Part model, mm, in its own coordinate system. A direction names the side the tool comes from. Round coordinates to 2 decimals unless told otherwise and drop trailing zeros. Write each loop counter-clockwise with the first axis right and the second up, starting at its lowest first coordinate (ties: lowest second). Pieces come first, ordered by that corner, then holes. Notation, with made-up numbers: M 3,61 L 25,61 A26 ccw 25,89 Z; hole C 63,-13 d6. An arc over 180 degrees is marked long. Use one line per item in the form item = value. Start each with the question number.
Item 1: Flat gauge pins, fed straight in: pin 1 Ø12 at (x, z) = (54.5, 4.5) entering from -Y; pin 2 Ø2 at (x, y) = (54, 2) entering from -Z (3 decimals); pin 3 Ø2 at (x, y) = (22.5, -13.5) entering from -Z. Where does each tip first touch, or does it go through?
Item 2: Probe L1, parallel to X at y = -23, z = -4; L2, parallel to X at y = -5, z = 13.5; L3, parallel to Z at x = 27, y = -2. List the from-to ranges inside material, lowest first.
Item 3: Which spindle directions (+Z, -Z, +X, -X, +Y, -Y) get a long thin tool onto all of the face, cutting with end or side? Do faces 1 (the face through (110, 0, 3)), 2 (the face through (24.678, 23.846, -7.509)). Say none if no direction does.
Item 4: Cut at A-A, the plane x = 38. Give the cut face in (y, z).
Item 5: Cut at B-B, the plane x = 111.5. Give the cut face in (y, z), then the cut area to 3 significant figures.
Autodesk Inventor part; units mm, degrees
ref_plane "YZ Plane" through (0, 0, 0) normal (1, 0, 0) x (0, 1, 0)
ref_plane "XZ Plane" through (0, 0, 0) normal (0, 1, 0) x (-1, 0, 0)
ref_plane "XY Plane" through (0, 0, 0) normal (0, 0, 1) x (1, 0, 0)
sketch "草图1" plane through (0, 0, 0) normal (1, 0, 0) x (0, 1, 0)
  circle A0 centre (0, 0) radius 25
  dimension "d0" = 50
extrude "拉伸1" add sketch "草图1" along normal blind 50
sketch "草图2" plane through (50, 0, 0) normal (1, 0, 0) x (0, 0, -1)
  circle A0 centre (0, 0) radius 20
  dimension "d3" = 40
extrude "拉伸2" add sketch "草图2" along normal blind 40
sketch "草图3" plane through (90, 0, 0) normal (1, 0, 0) x (0, 0, -1)
  circle A0 centre (0, 0) radius 3
  dimension "d6" = 6
extrude "拉伸3" add sketch "草图3" along normal blind 40
fillet "圆角1" radius 2 1 edges at (130, 0, 3)
fillet "圆角2" radius 2 1 edges at (90, 0, 20)
fillet "圆角3" radius 2 2 edges at (50, -25, 0) (0, -25, 0)
fillet "圆角3" radius 2 2 edges at (90, 0, 3) (50, 0, 20)
properties part number "马达"
Model answer:
q1.pin_1 = -24.7
q1.pin_2 = -19.975
q1.pin_3 = -21.65
q2.L1 = 0.03 to 49.97
q2.L2 = 0 to 90
q2.L3 = -24.92 to 24.92
q3.face_1 = +X
q3.face_2 = +X, -X
q4.outline = C 0,0 d50
q5.outline = C 0,0 d6
q5.area = 28.3 mm²
